Input: part model. Units: mm. Frame: model coordinates. A direction names the side the tool comes from. Coordinates: 2 decimals unless noted, no trailing zeros. Loops run counter-clockwise (first coordinate to the right, second up) from the corner with the lowest first, then second, coordinate; pieces in that order, holes last. Notation, with made-up numbers: (68.5, 14.5) - (78.5, 14.5) arc R20 cw to (78.5, 48.5) - close; hole circle Ø3 at (42.25, 16). An arc over 180 degrees is marked (long way). Use one line per item in the form item = value.
from build123d import *

# Parameters (mm, degrees)
F2_R     = 6
F3_DEPTH = 50


with BuildPart() as f1:
    # F0 (on Front) → F1 (revolve)
    with BuildSketch(Plane.XZ):
        Polygon((20, 5), (20, 0), (42.25, 0), (42.25, 4.2), (38.25, 4.2), (38.25, 9.2), (42.25, 9.2), (42.25, 24.5), (30, 24.5), (30, 10), (16, 10), (16, 5), align=None)
    revolve(axis=Axis((0, 0, 1.3315217948), (0, 0, -1)))


with BuildPart() as f3:
    # F2 (on Front) → F3 (new body, symmetric)
    with BuildSketch(Plane.XZ):
        with Locations((33.65, 15)):
            Circle(F2_R)
    extrude(amount=F3_DEPTH, both=True)


with BuildPart() as f1_1:
    add(f1.part)

    # F4: cut F3
    add(f3.part, mode=Mode.SUBTRACT)


solid = f1_1.part
Q1. Set-up query: faces 1 (the cylindrical face through (-4.336, 19.524, 2.465)), 2 (the flat face through (39, 0, 9.2)), 3 (the flat face through (-38, 6, 9.2)). Return all of +Z, -Z, +X, -X, +Y, -Y with unobstructed straight access to the full face (end or side cutting, diameter ignored); none if empty.
Check values:
face_1 = -Z
face_2 = +X
face_3 = none
Q2. Cut plane B-B, the plane y = 0. Return loops of the section in (x, z), then the cut area to 3 significant figures.
Check values:
outline = (-42.25, 0) - (-20, 0) - (-20, 5) - (-16, 5) - (-16, 10) - (-30, 10) - (-30, 24.5) - (-42.25, 24.5) - (-42.25, 9.2) - (-38.25, 9.2) - (-38.25, 4.2) - (-42.25, 4.2) - close; (16, 5) - (20, 5) - (20, 0) - (42.25, 0) - (42.25, 4.2) - (38.25, 4.2) - (38.25, 9.2) - (42.25, 9.2) - (42.25, 24.5) - (30, 24.5) - (30, 19.76) arc R6 cw (long way) to (30, 10.24) - (30, 10) - (16, 10) - close
area = 703 mm²
Q3. Cut plane D-D, the plane x = 33.65. Return loops of the section in (y, z).
Check values:
outline = (-25.55, 0) - (25.55, 0) - (25.55, 4.2) - (18.19, 4.2) - (18.19, 9) - (-18.19, 9) - (-18.19, 4.2) - (-25.55, 4.2) - close; (-25.55, 21) - (25.55, 21) - (25.55, 24.5) - (-25.55, 24.5) - close
Q4. Ray query, line 1 along Y through (x, z) = (0, 3.1); line 2 along X through (y, z) = (10.5, 17.75); line 3 along Z through (x, y) = (33.65, -9.5). Return the intervals inside material, ascending. Write a range as [from, to].
Check values:
line_1 = [-42.25, -20], [20, 42.25]
line_2 = [-40.92, -28.1], [28.1, 28.32], [38.98, 40.92]
line_3 = [0, 9], [21, 24.5]
Q5. Pull-direction query (Y, two-part tool) for faces 4 (the cylindrical face through (-29.97, -1.32, 17.15)), 5 (the flat face through (-6, -38, 4.2)), 6 (the flat face through (8.98, -13.43, 5)), 7 (the cylindrical face through (-30.354, 23.275, 6.735)); classes: pulls with the +Y half, pulls with the -Y half, needs draft (parallel to the pull), parting line crosses it, or undercut.
Check values:
face_4 = undercut
face_5 = needs draft
face_6 = undercut
face_7 = parting line crosses it
Q6. First-contact query: P1, Ø10, axis at y = 14, z = 10, coming from the -X side; P2, Ø10, axis at x = 6, z = 3.5, coming from the +Y side; P3, Ø8, axis at x = -18.5, z = 4, coming from the +Y side. Flat tips, straight axial feed; report the tip coordinate or a pass-through.
Check values:
P1 = -41.28
P2 = 42.24
P3 = 39.68
Q7. Cut plane C-C, the plane z = 15. Return loops of the section in (x, y).
Check values:
outline = (27.65, -31.95) - (27.65, -11.64) arc R30 cw (long way) to (27.65, 11.64) - (27.65, 31.95) arc R42.25 ccw (long way) to start; (39.65, -14.59) arc R42.25 ccw to (39.65, 14.59) - close
Q8. Cut plane A-A, the plane x = 0. Return loops of the section in (y, z), then the cut area to 3 significant figures.
Check values:
outline = (-42.25, 0) - (-20, 0) - (-20, 5) - (-16, 5) - (-16, 10) - (-30, 10) - (-30, 24.5) - (-42.25, 24.5) - (-42.25, 9.2) - (-38.25, 9.2) - (-38.25, 4.2) - (-42.25, 4.2) - close; (16, 5) - (20, 5) - (20, 0) - (42.25, 0) - (42.25, 4.2) - (38.25, 4.2) - (38.25, 9.2) - (42.25, 9.2) - (42.25, 24.5) - (30, 24.5) - (30, 10) - (16, 10) - close
area = 800 mm²
